```python
from build123d import *

# Parameters (mm, degrees)
SKETCH1_W                       = 112
SKETCH1_H                       = 35.5
BOSS_EXTRUDE1_DEPTH             = 1
SKETCH2_W                       = 6
SKETCH2_H                       = 6
BOSS_EXTRUDE2_DEPTH             = 2
SKETCH3_R                       = 1.1
CUT_EXTRUDE1_DEPTH              = 4
SKETCH4_R                       = 2
CUT_EXTRUDE2_DEPTH              = 2
SKETCH5_W                       = 20
SKETCH5_H                       = 14
CUT_EXTRUDE3_DEPTH              = 4
CHAMFER1_SIZE                   = 0.4
CUT_EXTRUDE4_DEPTH              = 0.2
SKETCH7_W                       = 2.2
SKETCH7_H                       = 2.2
CUT_EXTRUDE5_DEPTH              = 0.2
MIRROR2_COPY_1_DEPTH            = 0.2
MIRROR2_COPY_2_SKETCH_W         = 2.2
MIRROR2_COPY_2_SKETCH_H         = 2.2
MIRROR2_COPY_2_DEPTH            = 0.2
SKETCH8_W                       = 0.4
SKETCH8_H                       = 35.5
CUT_EXTRUDE6_DEPTH              = 3
CUT_EXTRUDE6_DEPTH_BACK         = 2
SKIZZE1_W                       = 5.6
SKIZZE1_H                       = 23.5
AUFSATZ_LINEAR_AUSTRAGEN1_DEPTH = 2


with BuildPart() as part:
    # Sketch1 → Boss-Extrude1 (new body)
    with BuildSketch(Plane.XY):
        Rectangle(SKETCH1_W, SKETCH1_H)
    extrude(amount=BOSS_EXTRUDE1_DEPTH)

    # Sketch2 → Boss-Extrude2 (add)
    with BuildSketch(Plane.XY.offset(1)):
        with Locations((-53, 14.75)):
            Rectangle(SKETCH2_W, SKETCH2_H)
        with Locations((-53, -14.75)):
            Rectangle(SKETCH2_W, SKETCH2_H)
        with Locations((53, -14.75)):
            Rectangle(SKETCH2_W, SKETCH2_H)
        with Locations((53, 14.75)):
            Rectangle(SKETCH2_W, SKETCH2_H)
    extrude(amount=BOSS_EXTRUDE2_DEPTH)

    # Sketch3 → Cut-Extrude1 (cut, through all)
    with BuildSketch(Plane.XY.offset(3)):
        with Locations((-53, 14.75)):
            Circle(SKETCH3_R)
        with Locations((-53, -14.75)):
            Circle(SKETCH3_R)
        with Locations((53, -14.75)):
            Circle(SKETCH3_R)
        with Locations((53, 14.75)):
            Circle(SKETCH3_R)
    extrude(amount=-CUT_EXTRUDE1_DEPTH, mode=Mode.SUBTRACT)

    # Sketch4 → Cut-Extrude2 (cut)
    with BuildSketch(Plane(origin=(0, 0, 0), x_dir=(-1, 0, 0), z_dir=(0, 0, -1))):
        with Locations((-53, 14.75)):
            Circle(SKETCH4_R)
        with Locations((-53, -14.75)):
            Circle(SKETCH4_R)
        with Locations((53, 14.75)):
            Circle(SKETCH4_R)
        with Locations((53, -14.75)):
            Circle(SKETCH4_R)
    extrude(amount=-CUT_EXTRUDE2_DEPTH, mode=Mode.SUBTRACT)

    # Sketch5 → Cut-Extrude3 (cut, through all)
    with BuildSketch(Plane(origin=(0, 0, 0), x_dir=(-1, 0, 0), z_dir=(0, 0, -1))):
        with Locations((29.95, 6.75)):
            Rectangle(SKETCH5_W, SKETCH5_H)
    extrude(amount=-CUT_EXTRUDE3_DEPTH, mode=Mode.SUBTRACT)

    # Chamfer1
    chamfer1_edges = [part.edges().sort_by_distance(p)[0] for p in [
        (-39.95, 6.75, 0),
        (-29.95, 13.75, 0),
        (-19.95, 6.75, 0),
        (-29.95, -0.25, 0),
    ]]
    chamfer(chamfer1_edges, length=CHAMFER1_SIZE)

    # Sketch6 → Cut-Extrude4 (cut)
    with BuildSketch(Plane(origin=(0, 0, 2), x_dir=(-1, 0, 0), z_dir=(0, 0, -1))):
        with BuildLine():
            Line((-54.1, 13.079670691), (-54.1, 16.420329309))
            ThreePointArc((-54.1, 16.420329309), (-53, 16.75), (-51.9, 16.420329309))
            Line((-51.9, 16.420329309), (-51.9, 13.079670691))
            ThreePointArc((-51.9, 13.079670691), (-53, 12.75), (-54.1, 13.079670691))
        make_face()
    cut_extrude4 = extrude(amount=-CUT_EXTRUDE4_DEPTH, mode=Mode.SUBTRACT)

    # Sketch7 → Cut-Extrude5 (cut)
    with BuildSketch(Plane(origin=(0, 0, 2.2), x_dir=(-1, 0, 0), z_dir=(0, 0, -1))):
        with Locations((-53, 14.75)):
            Rectangle(SKETCH7_W, SKETCH7_H)
    cut_extrude5 = extrude(amount=-CUT_EXTRUDE5_DEPTH, mode=Mode.SUBTRACT)

    # Mirror1: Cut-Extrude4, Cut-Extrude5 across plane
    add(cut_extrude4.mirror(Plane(origin=(0, 0, 0), x_dir=(0, 0, 1), z_dir=(1, 0, 0))), mode=Mode.SUBTRACT)
    add(cut_extrude5.mirror(Plane(origin=(0, 0, 0), x_dir=(0, 0, 1), z_dir=(1, 0, 0))), mode=Mode.SUBTRACT)

    # Mirror2: Cut-Extrude4, Cut-Extrude5 across plane
    add(cut_extrude4.mirror(Plane.ZX), mode=Mode.SUBTRACT)
    add(cut_extrude5.mirror(Plane.ZX), mode=Mode.SUBTRACT)

    # Mirror2 copy 1 sketch → Mirror2 copy 1 (cut)
    with BuildSketch(Plane(origin=(0, 0, 2), x_dir=(1, 0, 0), z_dir=(0, 0, -1))):
        with BuildLine():
            Line((-54.1, 13.079670691), (-54.1, 16.420329309))
            ThreePointArc((-54.1, 16.420329309), (-53, 16.75), (-51.9, 16.420329309))
            Line((-51.9, 16.420329309), (-51.9, 13.079670691))
            ThreePointArc((-51.9, 13.079670691), (-53, 12.75), (-54.1, 13.079670691))
        make_face()
    extrude(amount=-MIRROR2_COPY_1_DEPTH, mode=Mode.SUBTRACT)

    # Mirror2 copy 2 sketch → Mirror2 copy 2 (cut)
    with BuildSketch(Plane(origin=(0, 0, 2.2), x_dir=(1, 0, 0), z_dir=(0, 0, -1))):
        with Locations((-53, 14.75)):
            Rectangle(MIRROR2_COPY_2_SKETCH_W, MIRROR2_COPY_2_SKETCH_H)
    extrude(amount=-MIRROR2_COPY_2_DEPTH, mode=Mode.SUBTRACT)

    # Sketch8 → Cut-Extrude6 (cut, two sides)
    with BuildSketch(Plane.XY.offset(1)) as cut_extrude6_sk:
        with Locations((-55.8, 0)):
            Rectangle(SKETCH8_W, SKETCH8_H)
        with Locations((55.8, 0)):
            Rectangle(SKETCH8_W, SKETCH8_H)
    extrude(amount=CUT_EXTRUDE6_DEPTH, mode=Mode.SUBTRACT)
    extrude(cut_extrude6_sk.sketch, amount=-CUT_EXTRUDE6_DEPTH_BACK, mode=Mode.SUBTRACT)

    # Skizze1 → Aufsatz-Linear austragen1 (add)
    with BuildSketch(Plane.XY.offset(1)):
        Polygon((50, -8.156810447), (-50, -8.156810447), (-50, -11.75), (-50, -17.75), (50, -17.75), (50, -11.75), align=None)
        with Locations((-52.8, 0)):
            Rectangle(SKIZZE1_W, SKIZZE1_H)
        with Locations((52.8, 0)):
            Rectangle(SKIZZE1_W, SKIZZE1_H)
    extrude(amount=AUFSATZ_LINEAR_AUSTRAGEN1_DEPTH)


solid = part.part
```
Source: CAD feature listing. Evaluate the final solid. Frame: model axes, mm. A direction names the side the tool comes from. Round coordinates to 2 decimals unless told otherwise and drop trailing zeros. Loops run counter-clockwise (first coordinate to the right, second up) from the corner with the lowest first, then second, coordinate; pieces in that order, holes last.
(1) Pull-direction query (X, two-part tool) for faces 3 (the cylindrical face through (52.13, -15.42, 2.7)), 4 (the flat face through (-55.6, 0, 1)), 5 (the flat face through (-1, 5, 1)), 6 (the flat face through (0, -9, 3)); classes: +X half, -X half, draft (parallel to the pull), parting line (faces both ways), or undercut.
From the geometry:
face 3: undercut
face 4: -X half
face 5: undercut
face 6: draft
(2) Material intervals for probe 1 along Y at (x, z) = (-53, 2.6); probe 2 along Y at (x, z) = (-53, 0.85); probe 3 along X at (y, z) = (-14.75, 2.65), sorted ascending.
From the geometry:
probe 1: y = -17.75 to -15.85, -13.65 to 13.65, 15.85 to 17.75
probe 2: y = -17.75 to -16.75, -12.75 to 12.75, 16.75 to 17.75
probe 3: x = -55.6 to -54.1, -51.9 to 51.9, 54.1 to 55.6
(3) Access query for faces 1 (the cylindrical face through (-53.87, 14.08, 2.7)), 2 (the flat face through (1, -8.157, 2)). Directions: +Z, -Z, +X, -X, +Y, -Y. A direction counts if a zero-diameter tool reaches every point of the face in a straight line with its end or side. Return the directions, or none.
From the geometry:
face 1: +Z, -Z
face 2: +Z, +Y
(4) Section query C-C (y = -6.5). Output: boundary loops of the cut face in (x, z), and give its area (3 significant figures).
From the geometry:
outline: (-55.6, 0) - (55.6, 0) - (55.6, 3) - (50, 3) - (50, 1) - (-50, 1) - (-50, 3) - (-55.6, 3) - close
area: 134 mm2
(5) Section query B-B (x = -18.5). Output: boundary loops of the cut face in (y, z), and give its area (3 significant figures).
From the geometry:
outline: (-17.75, 0) - (17.75, 0) - (17.75, 1) - (-8.16, 1) - (-8.16, 3) - (-17.75, 3) - close
area: 54.7 mm2
(6) Section query A-A (y = 11.5). Output: boundary loops of the cut face in (x, z).
From the geometry:
outline: (-55.6, 0) - (-40.35, 0) - (-39.95, 0.4) - (-39.95, 1) - (-50, 1) - (-50, 3) - (-55.6, 3) - close; (-19.95, 0.4) - (-19.55, 0) - (55.6, 0) - (55.6, 3) - (50, 3) - (50, 1) - (-19.95, 1) - close
(7) Contact query for flat-ended pins moving along their axis: pin 1 Ø0.9 at (x, y) = (-52.5, -15.5) entering from -Z; pin 2 Ø0.7 at (x, y) = (-54.5, -15) entering from -Z. Output: stop coordinate, or through.
From the geometry:
pin 1: stops at z = 2.2
pin 2: stops at z = 2
